Source: CAD feature listing. Evaluate the final solid. Frame: model axes, mm. Give positions to 0.01 mm unless a question says otherwise; leave off trailing zeros. Order: outer loops, then holes, each group sorted by start corner. A loop starts at its lowest first (then second) coordinate and runs counter-clockwise, first axis right, second up. Notation, with made-up numbers: (-12, 59.25) - (-5, 59.25) arc R14 cw to (-5, 74.25) - close; hole circle Ø11 at (74.5, 82.5). An arc over 180 degrees is marked (long way). Use CSV: the item, a comma, the result in double quotes.
```python
from build123d import *

# Parameters (mm, degrees)
F0_W     = 196.844284
F0_H     = 77.783168
F0_R     = 30.48
F1_DEPTH = 12.7


with BuildPart() as f1:
    # F0 (on Front) → F1 (new body)
    with BuildSketch(Plane.XZ):
        with Locations((63.5, 0)):
            Rectangle(F0_W, F0_H)
        Circle(F0_R, mode=Mode.SUBTRACT)
        with Locations((63.5, 0)):
            Circle(F0_R, mode=Mode.SUBTRACT)
        with Locations((127, 0)):
            Circle(F0_R, mode=Mode.SUBTRACT)
    extrude(amount=-F1_DEPTH)


solid = f1.part
```
Item 1: Section D-D on x = 47. Return the cut outline in (y, z).
Filled in:
outline,"(0, -38.89) - (12.7, -38.89) - (12.7, -25.63) - (0, -25.63) - close; (0, 25.63) - (12.7, 25.63) - (12.7, 38.89) - (0, 38.89) - close"
Item 2: Section B-B on z = 0. Return the cut outline in (x, y).
Filled in:
outline,"(-34.92, 0) - (-30.48, 0) - (-30.48, 12.7) - (-34.92, 12.7) - close; (30.48, 0) - (33.02, 0) - (33.02, 12.7) - (30.48, 12.7) - close; (93.98, 0) - (96.52, 0) - (96.52, 12.7) - (93.98, 12.7) - close; (157.48, 0) - (161.92, 0) - (161.92, 12.7) - (157.48, 12.7) - close"
Item 3: Section A-A on x = 0. Return the cut outline in (y, z).
Filled in:
outline,"(0, -38.89) - (12.7, -38.89) - (12.7, -30.48) - (0, -30.48) - close; (0, 30.48) - (12.7, 30.48) - (12.7, 38.89) - (0, 38.89) - close"
Item 4: Section C-C on y = 3.5. Return the cut outline in (x, z), then the cut area to 3 significant figures.
Filled in:
outline,"(-34.92, -38.89) - (161.92, -38.89) - (161.92, 38.89) - (-34.92, 38.89) - close; hole circle Ø60.96 at (0, 0); hole circle Ø60.96 at (63.5, 0); hole circle Ø60.96 at (127, 0)"
area,"6,560 mm2"
Item 5: Material intervals for line 1 (X direction, y = 11.5, z = -24); line 2 (Z direction, x = 63.5, y = 7.75); line 3 (X direction, y = 3, z = -3), sorted ascending. Write a range as from..to.
Filled in:
line 1,"x = -34.92..-18.79, 18.79..44.71, 82.29..108.21, 145.79..161.92"
line 2,"z = -38.89..-30.48, 30.48..38.89"
line 3,"x = -34.92..-30.33, 30.33..33.17, 93.83..96.67, 157.33..161.92"
Item 6: Mould query, pull axis X, two halves, no side actions, for faces 1 (the cylindrical face through (-6.607, 6.261, -29.755)), 2 (the flat face through (161.922, 6, -1)), 3 (the flat face through (-34.922, 6, -1)), 4 (the flat face through (40, 0, 26)). Classes: released by +X, released by -X, zero draft, split by the parting line, or undercut.
Filled in:
face 1,"undercut"
face 2,"released by +X"
face 3,"released by -X"
face 4,"zero draft"
